from build123d import *

# Parameters (mm, degrees)
F0_W     = 170
F0_H     = 80
F1_DEPTH = 2.5
F2_R     = 3.4
F2_R_2   = 10
F2_R_3   = 2.75
F3_DEPTH = 5
F4_R     = 3


with BuildPart() as f1:
    # F0 (on Top) → F1 (new body, symmetric)
    with BuildSketch(Plane.XY):
        Rectangle(F0_W, F0_H)
    extrude(amount=F1_DEPTH, both=True)

    # F2 (on face) → F3 (cut)
    with BuildSketch(Plane.XY.offset(2.5)):
        with Locations((40, 25)):
            Circle(F2_R)
        with Locations((70, 25)):
            Circle(F2_R)
        with Locations((-40, 25)):
            Circle(F2_R)
        with Locations((-70, 25)):
            Circle(F2_R)
        with Locations((0, -20)):
            Circle(F2_R_2)
        with Locations((-23, -2)):
            Circle(F2_R_3)
        with Locations((-23, -20)):
            Circle(F2_R_3)
        with Locations((23, -2)):
            Circle(F2_R_3)
        with Locations((23, -20)):
            Circle(F2_R_3)
    extrude(amount=-F3_DEPTH, mode=Mode.SUBTRACT)

    # F4
    f4_edges = [f1.edges().sort_by_distance(p)[0] for p in [
        (-85, -40, 0),
        (85, -40, 0),
        (-85, 40, 0),
        (85, 40, 0),
    ]]
    fillet(f4_edges, radius=F4_R)


solid = f1.part
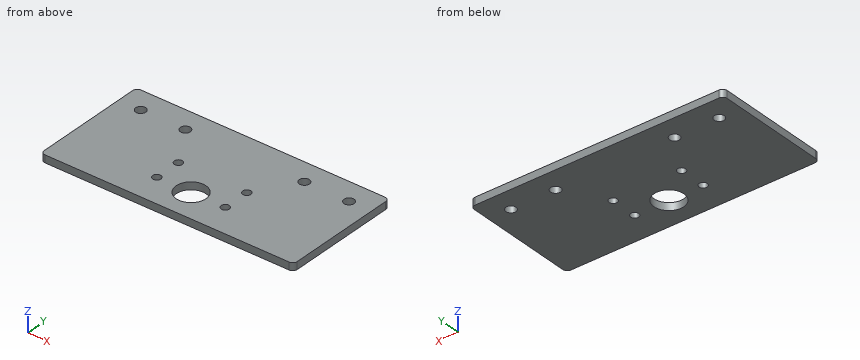
Verification items for the finished model (mm, model axes). Give positions to 0.01 mm unless a question says otherwise; leave off trailing zeros. Loops run counter-clockwise (first coordinate to the right, second up) from the corner with the lowest first, then second, coordinate; pieces in that order, holes last. Notation, with made-up numbers: (88, -10.75) - (118, -10.75) arc R23 cw to (118, 25.25) - close; hole circle Ø10 at (56, 26). An arc over 180 degrees is marked (long way). Write item = value, one per line. Start each with the question number.
Q1. Cross-section at C-C, the plane z = -1.15. State how many separate pieces and enclosed holes the cut face has, and give its area (3 significant figures).
Q2. Cross-section at A-A, the plane y = -2. Enter the section's corners in (x, z).
Q3. Cross-section at D-D, the plane y = -20. Enter the section's corners in (x, z).
Q4. Thickness scan on line 1 (X direction, y = 24.5, z = -0.85); line 2 (Y direction, x = 23, z = -0.65); line 3 (Y direction, x = 40, z = -0.2). Record the ranges inside material, lowest first.
Q5. Cross-section at B-B, the plane x = 40. Enter the section's corners in (y, z).
Answer key:
q1.separate_pieces = 1
q1.enclosed_holes = 9
q1.area = 13,000 mm^2
q2.outline = (-85, -2.5) - (-25.75, -2.5) - (-25.75, 2.5) - (-85, 2.5) - close; (-20.25, -2.5) - (20.25, -2.5) - (20.25, 2.5) - (-20.25, 2.5) - close; (25.75, -2.5) - (85, -2.5) - (85, 2.5) - (25.75, 2.5) - close
q3.outline = (-85, -2.5) - (-25.75, -2.5) - (-25.75, 2.5) - (-85, 2.5) - close; (-20.25, -2.5) - (-10, -2.5) - (-10, 2.5) - (-20.25, 2.5) - close; (10, -2.5) - (20.25, -2.5) - (20.25, 2.5) - (10, 2.5) - close; (25.75, -2.5) - (85, -2.5) - (85, 2.5) - (25.75, 2.5) - close
q4.line_1 = -85 to -73.36, -66.64 to -43.36, -36.64 to 36.64, 43.36 to 66.64, 73.36 to 85
q4.line_2 = -40 to -22.75, -17.25 to -4.75, 0.75 to 40
q4.line_3 = -40 to 21.6, 28.4 to 40
q5.outline = (-40, -2.5) - (21.6, -2.5) - (21.6, 2.5) - (-40, 2.5) - close; (28.4, -2.5) - (40, -2.5) - (40, 2.5) - (28.4, 2.5) - close
